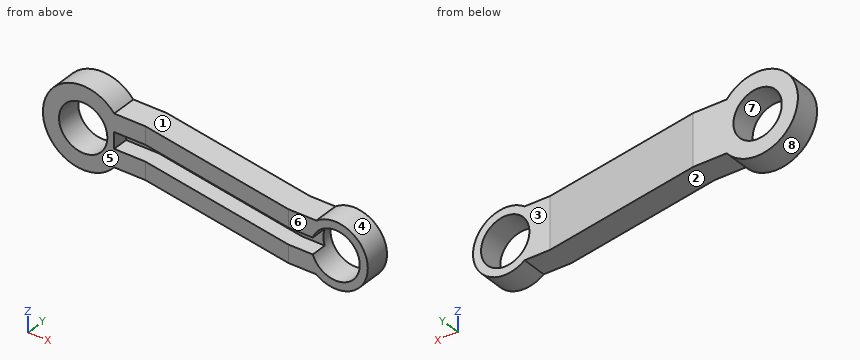
```python
from build123d import *

# Parameters (mm, degrees)
F0_R     = 7.5
F1_DEPTH = 25
F3_DEPTH = 12.5
F5_DEPTH = 2.5


with BuildPart() as f1:
    # F0 (on Front) → F1 (new body)
    with BuildSketch(Plane.XZ):
        with BuildLine():
            ThreePointArc((9.6046863561, -8), (11.7539052968, -4.2539052968), (12.5, 0))
            ThreePointArc((12.5, 0), (11.7539052968, 4.2539052968), (9.6046863561, 8))
            ThreePointArc((9.6046863561, 8), (-12.5, 0), (9.6046863561, -8))
        make_face()
        Circle(F0_R, mode=Mode.SUBTRACT)
        with BuildLine():
            ThreePointArc((95, 0), (89.472135955, 8.94427191), (79, 8))
            ThreePointArc((79, 8), (75, 0), (79, -8))
            ThreePointArc((79, -8), (89.472135955, -8.94427191), (95, 0))
        make_face()
        with Locations((85, 0)):
            Circle(F0_R, mode=Mode.SUBTRACT)
        with BuildLine():
            ThreePointArc((9.6046863561, 8), (11.7539052968, 4.2539052968), (12.5, 0))
            ThreePointArc((12.5, 0), (11.7539052968, -4.2539052968), (9.6046863561, -8))
            Line((9.6046863561, -8), (79, -8))
            ThreePointArc((79, -8), (75, 0), (79, 8))
            Line((79, 8), (9.6046863561, 8))
        make_face()
    extrude(amount=F1_DEPTH)

    # F2 (on Top) → F3 (intersect, symmetric)
    with BuildSketch(Plane.XY):
        Polygon((20, 0), (-12.5, 0), (-12.5, -8), (19.3000906918, -8), (70.3416270684, -17), (95, -17), (95, -9), (71.0415363766, -9), align=None)
    extrude(amount=F3_DEPTH, both=True, mode=Mode.INTERSECT)

    # F4 (on Top) → F5 (cut, symmetric)
    with BuildSketch(Plane.XY):
        Polygon((9.6046863561, -3), (9.6046863561, -8), (19.3000906918, -8), (21.884876116, -8.4557674096), (67.7568416441, -16.5442325904), (70.3416270684, -17), (79, -17), (79, -12), (70.779070386, -12), (19.7375340094, -3), align=None)
    extrude(amount=F5_DEPTH, both=True, mode=Mode.SUBTRACT)


solid = f1.part
```
Build history of the part. All positions in model axes, mm. Face numbers are marked on the shaded views. A direction names the side the tool comes from. Give positions to 0.01 mm unless a question says otherwise; leave off trailing zeros. Order: outer loops, then holes, each group sorted by start corner. A loop starts at its lowest first (then second) coordinate and runs counter-clockwise, first axis right, second up. Notation, with made-up numbers: M 28.5,-5.5 L 65.5,-5.5 A23 cw 65.5,32.5 Z; hole C -25,-23.75 d2. An arc over 180 degrees is marked long. Return JSON: item names as keys, results as strings.
Q1. Band-saw the part on C-C (y = -6.25). Give the cut face in (x, z).
Answer list:
{"outline": "M 9.6,-8 L 55.45,-8 L 55.45,8 L 9.6,8 A12.5 ccw long Z; hole C 0,0 d15; hole M 9.6,-2.5 L 38.17,-2.5 L 38.17,2.5 L 9.6,2.5 Z"}
Q2. 3-axis set-ups, long thin cutter, end or side, ignore diameter. For the marked faces 1, 2, 3, 4 and 5: which of +Z, -Z, +X, -X, +Y, -Y reach the whole face in a straight line?
Answer list:
{"face 1": "+Z, +Y, -Y", "face 2": "-Z, +Y, -Y", "face 3": "+Z, -Z, +X, +Y", "face 4": "+Y, -Y", "face 5": "+Z, -Z, -X, -Y"}
Q3. Band-saw the part on D-D (x = 11). Give the cut face in (y, z).
Answer list:
{"outline": "M -8,-8 L 0,-8 L 0,8 L -8,8 L -8,2.5 L -3,2.5 L -3,-2.5 L -8,-2.5 Z"}
Q4. Flat gauge pins, fed straight in: pin 1 (3 mm diameter, centred on x = 71, y = -13, fed in from +Z); pin 2 (4 mm diameter, centred on x = 81.5, y = -9.5, fed in from +Z); pin 3 (2 mm diameter, centred on x = 1, z = 9.5, fed in from -Y); pin 4 (12 mm diameter, centred on x = 0, z = 0, fed in from +Y). Where does each tip first touch, or does it go through?
Answer list:
{"pin 1": "stops at z = 8", "pin 2": "stops at z = 9.89", "pin 3": "stops at y = -8", "pin 4": "passes through"}
Q5. Wall check: probe 1 along Z at (x, y) = (67, -15.5); probe 2 along Z at (x, y) = (85, -11); probe 3 along Y at (x, z) = (13, -5.25). Give the ranges that are in metal, low to high. Write a range as from..to.
Answer list:
{"probe 1": "z = -8..-2.5, 2.5..8", "probe 2": "z = -10..-7.5, 7.5..10", "probe 3": "y = -8..0"}
Q6. Band-saw the part on B-B (z = 0). Give the cut face in (x, y).
Answer list:
{"outline": "M -12.5,-8 L -7.5,-8 L -7.5,0 L -12.5,0 Z; M 7.5,-8 L 9.6,-8 L 9.6,-3 L 19.74,-3 L 70.78,-12 L 77.5,-12 L 77.5,-9 L 71.04,-9 L 20,0 L 7.5,0 Z; M 92.5,-17 L 95,-17 L 95,-9 L 92.5,-9 Z"}
Q7. Band-saw the part on A-A (x = 85). Give the cut face in (y, z).
Answer list:
{"outline": "M -17,-10 L -9,-10 L -9,-7.5 L -17,-7.5 Z; M -17,7.5 L -9,7.5 L -9,10 L -17,10 Z"}
Q8. Two-plate mould, pull along Z, no slides. Class the marked faces 6, 7 and 8: pulls with the +Z half, pulls with the -Z half, needs draft (parallel to the pull), parting line crosses it, or undercut.
Answer list:
{"face 6": "needs draft", "face 7": "undercut", "face 8": "parting line crosses it"}
